Input: part model. Units: mm. Frame: model coordinates. Face numbers are marked on the shaded views. A direction names the side the tool comes from. Round coordinates to 2 decimals unless told otherwise and drop trailing zeros. Loops run counter-clockwise (first coordinate to the right, second up) from the corner with the lowest first, then second, coordinate; pieces in that order, holes last. Notation, with made-up numbers: (25, 4) -> (67, 4) arc R33 ccw to (67, 33) -> close; hole circle Ø7 at (-34.75, -21.75). An arc over 180 degrees is marked (long way). Answer in a Markdown table with one row per item. Add a question column.
Q1. Section D-D, the plane z = 31. Output: boundary loops of the cut face in (x, y).
Q2. Section C-C, the plane y = -15.5. Output: boundary loops of the cut face in (x, z), and give its area (3 significant figures).
Q3. Section A-A, the plane z = 23.5. Output: boundary loops of the cut face in (x, y).
Q4. Ray query, L1, parallel to Y at x = 52.75, z = 17.25; L2, parallel to X at y = 3.5, z = 22.25; L3, parallel to Y at x = 74, z = 27. Return the intervals inside material, ascending. Write a range as from..to.
Q5. Reachability of the marked faces 1, 2 and 3 from +Z, -Z, +X, -X, +Y, -Y: full face, straight path, thin tool, end or side. Return the list, or none.
Q6. Section B-B, the plane x = 52.75. Give the number of separate pieces and of enclosed holes in the cut face, and give its area (3 significant figures).
Q7. Pin query (flat end, axial travel): pin 1 (4 mm diameter, centred on y = 10, z = 18.5, fed in from +X); pin 2 (3 mm diameter, centred on y = -15, z = 24, fed in from -X); pin 3 (3 mm diameter, centred on x = 53.5, z = -0.5, fed in from -Y); pin 4 (1 mm diameter, centred on y = -14, z = 3, fed in from -X). Return the tip coordinate at first contact, or that it passes through.
Q8. Mould query, pull axis Z, two halves, no side actions, for the marked faces 4, 5 and 6. Classes: pulls with the +Z half, pulls with the -Z half, needs draft (parallel to the pull), parting line crosses it, or undercut.
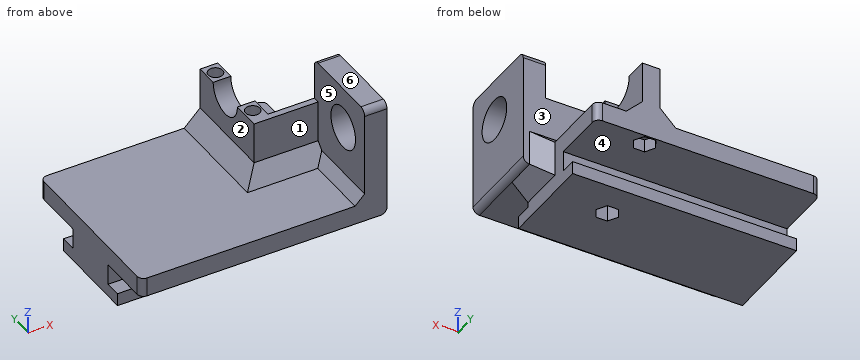
Autodesk Inventor part; units mm, degrees
ref_plane "YZ Plane" through (0, 0, 0) normal (1, 0, 0) x (0, 1, 0)
ref_plane "XZ Plane" through (0, 0, 0) normal (0, 1, 0) x (-1, 0, 0)
ref_plane "XY Plane" through (0, 0, 0) normal (0, 0, 1) x (1, 0, 0)
sketch "Sketch2" plane through (0, 0, 0) normal (1, 0, 0) x (0, 1, 0)
  line L0 (-19.9252, 0) -> (19.9252, 0)
  line L1 (0, -28.9507) -> (0, 28.9507)
  line L2 (14.5, -7.25) -> (-14.5, -7.25)
  line L3 (-14.5, -7.25) -> (-14.5, -3.25)
  line L4 (-9.5, -3.25) -> (-9.5, 3.25)
  line L5 (-27, 3.25) -> (-27, 9.25)
  line L6 (-27, 9.25) -> (27, 9.25)
  line L7 (14.5, -7.25) -> (14.5, -3.25)
  line L8 (9.5, -3.25) -> (9.5, 3.25)
  line L9 (27, 3.25) -> (27, 9.25)
  line L10 (-14.5, -3.25) -> (-9.5, -3.25)
  line L11 (9.5, -3.25) -> (14.5, -3.25)
  line L12 (27, 3.25) -> (9.5, 3.25)
  line L13 (-9.5, 3.25) -> (-27, 3.25)
  point P0 (0, 0)
  point P1 (0, 0)
  point P2 (9.5, 0)
  dimension "d4" = 14.5
  dimension "d8" = 27
  dimension "d9" = 9.5
  dimension "d10" = 4
  dimension "d11" = 6.5
  dimension "d12" = 6
extrude "Extrusion2" add sketch "Sketch2" along normal blind 70
sketch "Sketch3" plane through (0, -27, 9.25) normal (0, 0, 1) x (1, 0, 0)
  line L0 (0, 0) -> (70, 0)
  line L1 (0, 54) -> (70, 54)
  line L2 (50, 27) -> (50, 54)
  line L3 (50, 54) -> (55.5, 54)
  line L4 (55.5, 54) -> (55.5, 27)
  line L5 (70, 54) -> (70, 0)
  line L6 (50, 27) -> (55.5, 27)
  point P0 (0, 27)
  dimension "d15" = 20
  dimension "d16" = 5.5
  dimension "d43" = 27
  dimension "d44" = 27
extrude "Extrusion3" add sketch "Sketch3" along normal blind 18
sketch "Sketch7" plane through (0, -27, 3.25) normal (0, 0, -1) x (-1, 0, 0)
  line L0 (0, 0) -> (70, 0)
  line L1 (-70, 0) -> (-77, 0)
  line L2 (-77, 0) -> (-77, 27)
  line L3 (-77, 27) -> (-70, 27)
  line L4 (-70, 27) -> (-70, 0)
  line L5 (70, 54) -> (70, 0)
  line L6 (-70, 0) -> (-70, 17.5)
  point P0 (0, 27)
  dimension "d45" = 7
  dimension "d50" = 0
extrude "Extrusion6" add sketch "Sketch7" against normal blind 37
sketch "Sketch9" plane through (50, 0, 9.25) normal (-1, 0, 0) x (0, 0, 1)
  line L0 (18, 27) -> (18, 0)
  line L1 (0, -27) -> (31, -27)
  point P0 (-9.25, 0)
  point P1 (18, 13.5)
hole "Hole2" at (50, 13.5, 27.25) direction (1, 0, 0) diameter 13 end through all
sketch "Sketch10" plane through (0, -27, 27.25) normal (0, 0, 1) x (1, 0, 0)
  line L0 (55.5, 54) -> (50, 54)
  line L1 (50, 54) -> (50, 47)
  line L2 (55.5, 40.5) -> (50, 40.5)
  line L3 (50, 34) -> (50, 47)
  line L4 (70, 54) -> (70, 27)
  line L5 (55.5, 54) -> (70, 54)
  point P0 (0, 27)
  point P1 (52.75, 50.5)
  point P2 (52.75, 30.5)
  dimension "d99" = 20
  dimension "d100" = 13.5
  dimension "d101" = 2.75
  dimension "d102" = 3.5
  dimension "d103" = 2.75
  dimension "d104" = 23.5
hole "Hole3" at (52.75, 23.5, 27.25) at (52.75, 3.5, 27.25) direction (0, 0, -1) diameter 4.5 end through all
sketch "Sketch11" plane through (0, -14.5, -7.25) normal (0, 0, -1) x (-1, 0, 0)
  circle A0 centre (-52.75, 18) radius 2.25
  line L0 (-56.25, 18) -> (-54.5, 21.0311)
  line L1 (-54.5, 21.0311) -> (-51, 21.0311)
  line L2 (-51, 21.0311) -> (-49.25, 18)
  line L3 (-49.25, 18) -> (-51, 14.9689)
  line L4 (-51, 14.9689) -> (-54.5, 14.9689)
  line L5 (-54.5, 14.9689) -> (-56.25, 18)
  circle A1 centre (-52.75, 38) radius 2.25
  line L6 (-56.25, 38) -> (-54.5, 41.0311)
  line L7 (-54.5, 41.0311) -> (-51, 41.0311)
  line L8 (-51, 41.0311) -> (-49.25, 38)
  line L9 (-49.25, 38) -> (-51, 34.9689)
  line L10 (-51, 34.9689) -> (-54.5, 34.9689)
  line L11 (-54.5, 34.9689) -> (-56.25, 38)
  point P0 (0, 14.5)
  dimension "d71" = 7
  dimension "d74" = 7
extrude "Extrusion7" cut sketch "Sketch11" against normal blind 14.5
fillet "Fillet1" radius 2 6 edges at (73.5, 0, 40.25) (73.5, -27, 40.25) (70, 27, 6.25) (0, 27, 6.25) (0, -27, 6.25) (77, -13.5, 3.25)
sketch "Sketch13" plane through (50, 0, 9.25) normal (0, -1, 0) x (1, 0, 0)
  line L0 (27, -4) -> (27, 29)
  line L1 (0, 18) -> (27, 18)
  line L2 (27, 18) -> (27, 0)
  line L3 (27, 0) -> (0, 0)
  line L4 (0, 0) -> (0, 18)
  point P0 (-50, -9.25)
  point P1 (20, 0)
  dimension "d95" = 0
extrude "Extrusion9" add sketch "Sketch13" along normal blind 2
chamfer "Chamfer3" distance 5 angle 45 6 edges at (50, 12.5, 9.25) (55.5, 13.5, 9.25) (70, -4.75, 3.25) (70, 0, 6.25) (62.75, 0, 9.25) (60, -2, 9.25)
sketch "Sketch14" plane through (70, -25, 40.25) normal (-1, 0, 0) x (0, 0, 1)
  circle A0 centre (-13, 9.5) radius 9.5
  line L0 (-31, -2) -> (-2, -2)
  line L1 (0, 23) -> (0, 0)
  point P0 (-40.25, 25)
  point P1 (-26, -2)
  dimension "d85" = 19
  dimension "d86" = 11.5
  dimension "d94" = 13
hole "Hole4" at (70, -15.5, 27.25) direction (1, 0, 0) diameter 13.2 end through all
chamfer "Chamfer4" distance 3 angle 45 1 edges at (70, -17, 9.25)
properties part number "CarroXY - Hotend"
Answer block:
| question | item | result |
|---|---|---|
| 1 | outline | (70, -27) -> (77, -27) -> (77, -20.93) -> (70, -20.93) -> close; (70, -10.07) -> (77, -10.07) -> (77, 0) -> (70, 0) -> close |
| 2 | outline | (0, 3.25) -> (75, 3.25) arc R2 ccw to (77, 5.25) -> (77, 20.65) -> (70, 20.65) -> (70, 12.25) -> (67, 9.25) -> (0, 9.25) -> close; (70, 33.85) -> (77, 33.85) -> (77, 40.25) -> (70, 40.25) -> close |
| 2 | area | 590 mm^2 |
| 3 | outline | (50, -2) -> (70, -2) -> (70, -10.07) -> (77, -10.07) -> (77, 0) -> (55.5, 0) -> (55.5, 8.19) -> (50, 8.19) -> close; (50, 18.81) -> (55.5, 18.81) -> (55.5, 27) -> (50, 27) -> close; (70, -27) -> (77, -27) -> (77, -20.93) -> (70, -20.93) -> close; hole circle Ø4.5 at (52.75, 3.5); hole circle Ø4.5 at (52.75, 23.5) |
| 4 | L1 | -2..1.25, 5.75..21.25, 25.75..27 |
| 4 | L2 | 50..50.5, 55..55.5 |
| 4 | L3 | -27..-22.1, -8.9..0 |
| 5 | face 1 | +Z, -X, -Y |
| 5 | face 2 | +Z, -X, +Y, -Y |
| 5 | face 3 | +Z, +X, +Y |
| 6 | separate pieces | 3 |
| 6 | enclosed holes | 0 |
| 6 | area | 739 mm^2 |
| 7 | pin 1 | x = 55.5 |
| 7 | pin 2 | through |
| 7 | pin 3 | y = -9.5 |
| 7 | pin 4 | x = 0 |
| 8 | face 4 | undercut |
| 8 | face 5 | needs draft |
| 8 | face 6 | pulls with the +Z half |
